Input: part model. Units: mm. Frame: model coordinates. A direction names the side the tool comes from. Give positions to 0.01 mm unless a question says otherwise; leave off trailing zeros. Order: outer loops, then holes, each group sorted by start corner. A loop starts at its lowest first (then second) coordinate and runs counter-clockwise, first axis right, second up. Notation, with made-up numbers: (66, -2.5) - (80, -2.5) arc R29 ccw to (80, 33.5) - close; hole circle Ø4 at (7.25, 15). An arc over 180 degrees is marked (long way). Answer in a Markdown table with one row per item. Add a question column.
1. Section query C-C on x = 1.15. Return loops of the section in (y, z), and give its area (3 significant figures).
2. Section query D-D on z = 52. Return loops of the section in (x, y), and give its area (3 significant figures).
3. Contact query for flat-ended pins moving along their axis: pin 1 (1 mm diameter, centred on x = 4.5, z = 71.5, fed in from -Y); pin 2 (1.5 mm diameter, centred on x = 1.5, z = 82.5, fed in from +Y); pin 3 (2.5 mm diameter, centred on x = 2, z = 22, fed in from +Y). Output: stop coordinate, or through.
4. Mould query, pull axis Z, two halves, no side actions, for faces 6 (the face through (2, 22, 80)), 7 (the face through (2, 32.5, 2)), 8 (the face through (2.465, 24.966, 37.021)). Classes: released by +Z, released by -Z, zero draft, split by the parting line, or undercut.
5. Ray query, line 1 (Z direction, x = 1.75, y = 69.5); line 2 (Y direction, x = 1.9, z = 36.5); line 3 (Z direction, x = 1.6, y = 100.5). Return the intervals inside material, ascending. Write a range as [from, to].
6. Section query A-A on z = 36.5. Return loops of the section in (x, y).
7. Section query B-B on y = 21. Return loops of the section in (x, z), and give its area (3 significant figures).
8. Access query for faces 1 (the face through (2.465, 73.773, 38.993)), 2 (the face through (2, 115, 65)), 3 (the face through (2, 82.5, 3)), 4 (the face through (2, -2, 30)), 5 (the face through (2, -3, 50)). Directions: +Z, -Z, +X, -X, +Y, -Y. A direction counts if a zero-diameter tool reaches every point of the face in a straight line with its end or side. Return the directions, or none.
```python
from build123d import *

# Parameters (mm, degrees)
SKETCH_1_R      = 4
SKETCH_1_R_2    = 11.5
SKETCH_1_R_3    = 1.5
EXTRUDE_1_DEPTH = 5


with BuildPart() as part:
    # 草图1 → 凸台-拉伸1 (new body)
    with BuildSketch(Plane(origin=(0, 0, 0), x_dir=(0, 0, -1), z_dir=(1, 0, 0))):
        Polygon((-80, 70), (-80, 115), (-50, 115), (-50, 120), (-30, 120), (-30, 115), (-5, 115), (-5, 82.5), (0, 82.5), (0, 32.5), (-5, 32.5), (-5, 0), (-30, 0), (-30, -5), (-50, -5), (-50, 0), (-80, 0), (-80, 45), (-85, 45), (-85, 70), align=None)
        with Locations((-36.5, 21)):
            Circle(SKETCH_1_R, mode=Mode.SUBTRACT)
        with Locations((-36.5, 85)):
            Circle(SKETCH_1_R_2, mode=Mode.SUBTRACT)
        with Locations((-52, 100.5)):
            Circle(SKETCH_1_R_3, mode=Mode.SUBTRACT)
        with Locations((-21, 100.5)):
            Circle(SKETCH_1_R_3, mode=Mode.SUBTRACT)
        with Locations((-21, 69.5)):
            Circle(SKETCH_1_R_3, mode=Mode.SUBTRACT)
        with Locations((-52, 69.5)):
            Circle(SKETCH_1_R_3, mode=Mode.SUBTRACT)
    extrude(amount=EXTRUDE_1_DEPTH)


solid = part.part
```
Answer:
| question | item | result |
|---|---|---|
| 1 | outline | (-5, 30) - (0, 30) - (0, 5) - (32.5, 5) - (32.5, 0) - (82.5, 0) - (82.5, 5) - (115, 5) - (115, 30) - (120, 30) - (120, 50) - (115, 50) - (115, 80) - (70, 80) - (70, 85) - (45, 85) - (45, 80) - (0, 80) - (0, 50) - (-5, 50) - close; hole circle Ø8 at (21, 36.5); hole circle Ø3 at (69.5, 21); hole circle Ø3 at (69.5, 52); hole circle Ø23 at (85, 36.5); hole circle Ø3 at (100.5, 21); hole circle Ø3 at (100.5, 52) |
| 1 | area | 8,710 mm² |
| 2 | outline | (0, 0) - (5, 0) - (5, 68) - (0, 68) - close; (0, 71) - (5, 71) - (5, 99) - (0, 99) - close; (0, 102) - (5, 102) - (5, 115) - (0, 115) - close |
| 2 | area | 545 mm² |
| 3 | pin 1 | stops at y = 0 |
| 3 | pin 2 | stops at y = 70 |
| 3 | pin 3 | stops at y = 115 |
| 4 | face 6 | released by +Z |
| 4 | face 7 | zero draft |
| 4 | face 8 | undercut |
| 5 | line 1 | z = [0, 19.5], [22.5, 50.5], [53.5, 85] |
| 5 | line 2 | y = [-5, 17], [25, 73.5], [96.5, 120] |
| 5 | line 3 | z = [5, 19.5], [22.5, 50.5], [53.5, 80] |
| 6 | outline | (0, -5) - (5, -5) - (5, 17) - (0, 17) - close; (0, 25) - (5, 25) - (5, 73.5) - (0, 73.5) - close; (0, 96.5) - (5, 96.5) - (5, 120) - (0, 120) - close |
| 7 | outline | (0, 5) - (5, 5) - (5, 32.5) - (0, 32.5) - close; (0, 40.5) - (5, 40.5) - (5, 80) - (0, 80) - close |
| 7 | area | 335 mm² |
| 8 | face 1 | +X, -X |
| 8 | face 2 | +Z, +X, -X, +Y |
| 8 | face 3 | -Z, +X, -X, +Y |
| 8 | face 4 | -Z, +X, -X, -Y |
| 8 | face 5 | +Z, +X, -X, -Y |
